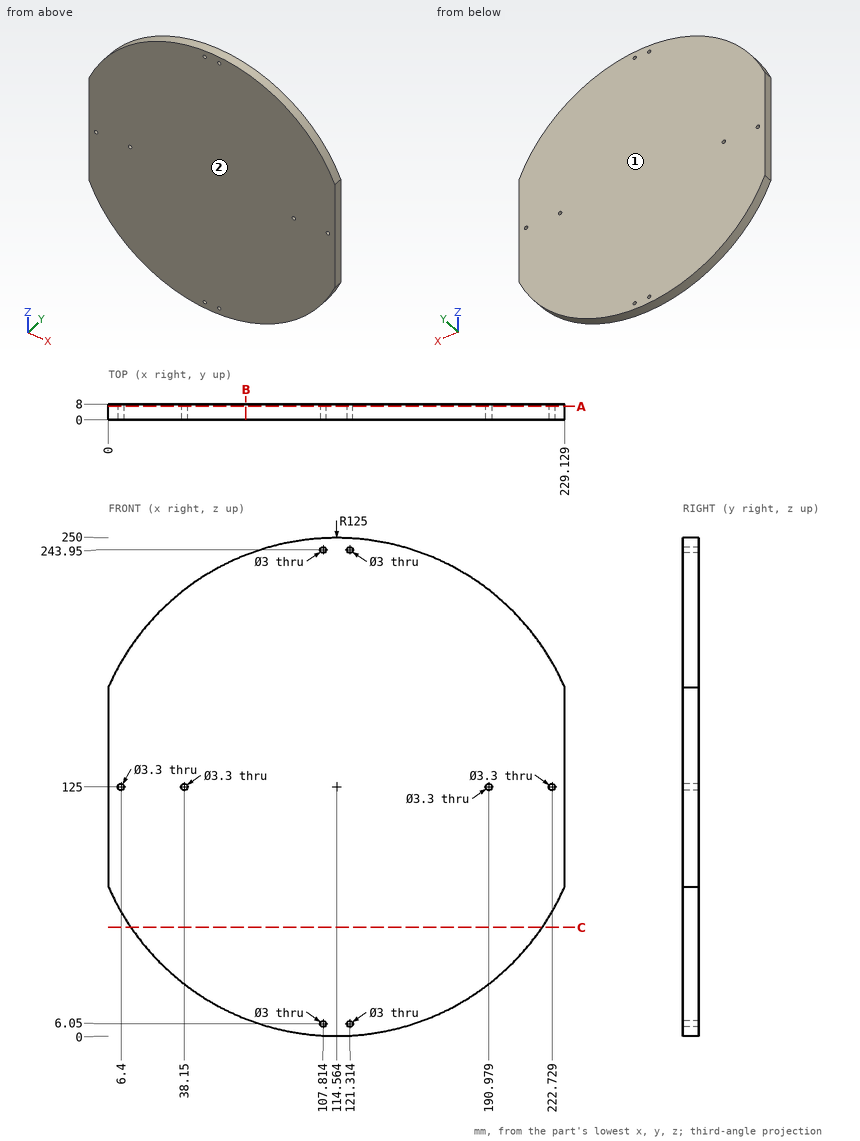
Source: three-view drawing plus pictorial views. Frame: mm from the lowest corner of the part. Give positions to 0.01 mm unless a question says otherwise; leave off trailing zeros. Order: outer loops, then holes, each group sorted by start corner. A loop starts at its lowest first (then second) coordinate and runs counter-clockwise, first axis right, second up. Notation, with made-up numbers: (37, 52) -> (70, 52) arc R20 ccw to (70, 82) -> close; hole circle Ø11 at (27.25, 40.25). An arc over 180 degrees is marked (long way). Write each question's results on one line, items separated by ' | '. Start each with the question number.
Item 1: Cut plane B-B on x = 69. Return the cut outline in (y, z).
Item 2: Mould query, pull axis Y, two halves, no side actions, for the marked faces 1 and 2. Classes: pulls with the +Y half, pulls with the -Y half, needs draft (parallel to the pull), parting line crosses it, or undercut.
Item 3: Cut plane C-C on z = 54.5. Return the cut outline in (x, y).
Item 4: Line query: line 1 (Z direction, x = 81, y = 1.75); line 2 (Z direction, x = 42, y = 1.25); line 3 (X direction, y = 1.5, z = 22.5). Output: solid intervals per line, ascending.
Item 5: Cut plane A-A on y = 6.75. Give the number of separate pieces and of enclosed holes in the cut face, then the cut area to 3 significant figures.
Item 6: Contact query for a flat-ended pin moving along its axis: P1, Ø1, axis at x = 140.5, y = 1, coming from the -Z side (1 decimal). Output: stop coordinate, or through.
Established:
1) outline: (0, 8.6) -> (8, 8.6) -> (8, 241.4) -> (0, 241.4) -> close
2) face 1: pulls with the +Y half | face 2: pulls with the -Y half
3) outline: (11.34, 0) -> (217.79, 0) -> (217.79, 8) -> (11.34, 8) -> close
4) line 1: 4.59 to 245.41 | line 2: 23.22 to 226.78 | line 3: 43.02 to 186.11
5) separate pieces: 1 | enclosed holes: 8 | area: 47,600 mm^2
6) P1: z = 2.6
